```python
from build123d import *

# Parameters (mm, degrees)
SKETCH_1_R         = 1.5
EXTRUDE_1052_DEPTH = 3
FILLET1_R          = 3
FILLET_1_R         = 2


with BuildPart() as part:
    # Эскиз1 → Extrude 1052 (new body)
    with BuildSketch(Plane.XY):
        with BuildLine():
            Line((-48.5, 5.5), (-48.5, -5.5))
            Line((-48.5, -5.5), (-15.5, -5.5))
            Line((-15.5, -5.5), (-5.5, -15.5))
            Line((-5.5, -15.5), (-5.5, -37))
            ThreePointArc((-5.5, -37), (-3.339392013, -40.233578364), (0.474873734, -39.474873734))
            Line((0.474873734, -39.474873734), (5.5, -34.449747468))
            Line((5.5, -34.449747468), (5.5, 5.5))
            Line((5.5, 5.5), (-48.5, 5.5))
        make_face()
        with Locations((-18.5, 0)):
            Circle(SKETCH_1_R, mode=Mode.SUBTRACT)
        with Locations((-41.5, 0)):
            Circle(SKETCH_1_R, mode=Mode.SUBTRACT)
        with Locations((-2, -13)):
            Circle(SKETCH_1_R, mode=Mode.SUBTRACT)
        with Locations((-2, -37)):
            Circle(SKETCH_1_R, mode=Mode.SUBTRACT)
    extrude(amount=EXTRUDE_1052_DEPTH)

    # Fillet1
    fillet1_edges = [part.edges().sort_by_distance(p)[0] for p in [
        (-15.5, -5.5, 1.5),
        (-5.5, -15.5, 1.5),
        (5.5, -34.449747468, 1.5),
        (5.5, 5.5, 1.5),
    ]]
    fillet(fillet1_edges, radius=FILLET1_R)

    # Скругление1
    fillet_1_edges = [part.edges().sort_by_distance(p)[0] for p in [
        (-48.5, 5.5, 1.5),
    ]]
    fillet(fillet_1_edges, radius=FILLET_1_R)


solid = part.part
```
The listing builds one solid part. Answer for the finished solid, in the listing's coordinates (mm). A direction names the side the tool comes from. Coordinates: 2 decimals unless noted, no trailing zeros. Write each loop counter-clockwise with the first axis right and the second up, starting at its lowest first coordinate (ties: lowest second). Pieces come first, ordered by that corner, then holes.
Q1. Find the intervals of material crossed by line 1 along Y through (x, z) = (-2, 1.75); line 2 along Y through (x, z) = (-18.5, 1.05); line 3 along Y through (x, z) = (-35.5, 1.75), in increasing order.
Returned:
line 1: y = -40.5 to -38.5, -35.5 to -14.5, -11.5 to 5.5
line 2: y = -5.5 to -1.5, 1.5 to 5.5
line 3: y = -5.5 to 5.5
Q2. Section A-A, the plane y = 0 is taken. Write down the section's boundary in (x, z), then the cut area to 3 significant figures.
Returned:
outline: (-48.5, 0) - (-43, 0) - (-43, 3) - (-48.5, 3) - close; (-40, 0) - (-20, 0) - (-20, 3) - (-40, 3) - close; (-17, 0) - (5.5, 0) - (5.5, 3) - (-17, 3) - close
area: 144 mm2
Q3. Section D-D, the plane y = -13 is taken. Write down the section's boundary in (x, z), then the cut area to 3 significant figures.
Returned:
outline: (-8, 0) - (-3.5, 0) - (-3.5, 3) - (-8, 3) - close; (-0.5, 0) - (5.5, 0) - (5.5, 3) - (-0.5, 3) - close
area: 31.5 mm2
Q4. Given P1, Ø0.9, axis at x = -27.5, z = 1, coming from the -Y side; P2, Ø1.5, axis at y = -31, z = 1, coming from the -X side, each flat-ended and moving along its own axis, determine where each tip first touches the part or whether it passes through.
Returned:
P1: stops at y = -5.5
P2: stops at x = -5.5
Q5. Section C-C, the plane x = -2 is taken. Write down the section's boundary in (y, z), then the cut area to 3 significant figures.
Returned:
outline: (-40.5, 0) - (-38.5, 0) - (-38.5, 3) - (-40.5, 3) - close; (-35.5, 0) - (-14.5, 0) - (-14.5, 3) - (-35.5, 3) - close; (-11.5, 0) - (5.5, 0) - (5.5, 3) - (-11.5, 3) - close
area: 120 mm2
Q6. Which of the six approach directions +Z, -Z, +X, -X, +Y, -Y give full straight-line access (tool end or side, diameter ignored) to faces 4 (the cylindrical face through (-43, 0, 1)), 5 (the flat face through (-33, -5.5, 1))?
Returned:
face 4: +Z, -Z
face 5: +Z, -Z, -X, -Y
Q7. The mould has two halves that part along Y. Classify faces 1 (the flat face through (-22, 5.5, 1)), 2 (the flat face through (-5.5, -27, 1)), 3 (the cylindrical face through (-20, 0, 1)): released by +Y, released by -Y, zero draft, split by the parting line, or undercut.
Returned:
face 1: released by +Y
face 2: zero draft
face 3: undercut
Q8. Section B-B, the plane x = -18.5 is taken. Write down the section's boundary in (y, z), then the cut area to 3 significant figures.
Returned:
outline: (-5.5, 0) - (-1.5, 0) - (-1.5, 3) - (-5.5, 3) - close; (1.5, 0) - (5.5, 0) - (5.5, 3) - (1.5, 3) - close
area: 24.0 mm2
